from build123d import *


with BuildPart() as part:
    # Sketch1 → Revolve-Thin1 (revolve)
    with BuildSketch(Plane.XY, mode=Mode.PRIVATE) as revolve_thin1_sk:
        Polygon((36.5, -1), (41.5, -1), (41.5, 1.36100674), (47.05164478, 3.931330757), (42.693587431, 6.382317526), (47.05164478, 8.400029378), (42.693587431, 10.851016147), (47.05164478, 12.868728), (42.693587431, 15.319714769), (47.05164478, 17.337426622), (42.693587431, 19.788413391), (47.05164478, 21.806125243), (42.693587431, 24.257112012), (47.05164478, 26.274823865), (42.693587431, 28.725810634), (47.05164478, 30.743522486), (41.5, 33.865787021), (41.5, 36.280890351), (36.5, 36.280890351), align=None)
        Polygon((37.5, 0), (40.5, 0), (40.5, 2), (44.858057349, 4.017711853), (40.5, 6.468698622), (44.858057349, 8.486410474), (40.5, 10.937397243), (44.858057349, 12.955109096), (40.5, 15.406095865), (44.858057349, 17.423807717), (40.5, 19.874794486), (44.858057349, 21.892506339), (40.5, 24.343493108), (44.858057349, 26.36120496), (40.5, 28.812191729), (44.858057349, 30.829903582), (40.5, 33.280890351), (40.5, 35.280890351), (37.5, 35.280890351), align=None, mode=Mode.SUBTRACT)
    revolve(revolve_thin1_sk.sketch.rotate(Axis((0, 76.319492769, 0), (0, -1, 0)), 90), axis=Axis((0, 76.319492769, 0), (0, -1, 0)))


solid = part.part
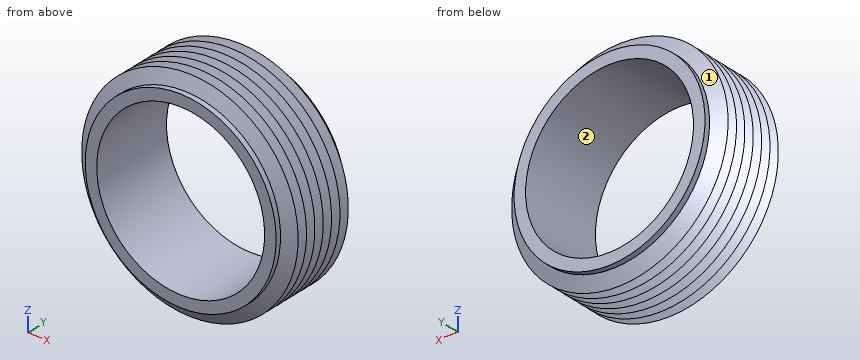
Source: CAD feature listing. Evaluate the final solid. Frame: model axes, mm. Face numbers are marked on the shaded views. Coordinates: 2 decimals unless noted, no trailing zeros. Use a Markdown table: item, result.
1) First-contact query: pin 1 Ø1 at (x, y) = (16, 4.5) entering from +Z; pin 2 Ø10 at (x, z) = (-29, 4) entering from -Y; pin 3 Ø3 at (y, z) = (4, 2) entering from +X. Flat tips, straight axial feed; report the tip coordinate or a pass-through.
Conclusion:
| item | result |
|---|---|
| pin 1 | stops at z = 44.13 |
| pin 2 | passes through |
| pin 3 | stops at x = 47.05 |
2) Mould query, pull axis X, two halves, no side actions, for the marked faces 1 and 2. Classes: pulls with the +X half, pulls with the -X half, needs draft (parallel to the pull), parting line crosses it, or undercut.
Conclusion:
| item | result |
|---|---|
| face 1 | parting line crosses it |
| face 2 | undercut |
3) Ray query, L1, parallel to Y at x = -20.5, z = 33; L2, parallel to X at y = 5, z = -1.5; L3, parallel to Z at x = 13.5, y = 17. Return the intervals inside material, ascending.
Conclusion:
| item | result |
|---|---|
| L1 | y = -1 to 0, 35.28 to 36.28 |
| L2 | x = -45.13 to -43.09, -37.47 to -36.47, 36.47 to 37.47, 43.09 to 45.13 |
| L3 | z = -44.31 to -41.82, -34.99 to -33.91, 33.91 to 34.99, 41.82 to 44.31 |
4) Section A-A, the plane z = 19.5. Give the number of separate pieces and of enclosed holes in the cut face, then the cut area to 3 significant figures.
Conclusion:
| item | result |
|---|---|
| separate pieces | 2 |
| enclosed holes | 2 |
| area | 270 mm^2 |
